from build123d import *

# Parameters (mm, degrees)
BOSS_EXTRUDE1_DEPTH  = 25.4
M3_CLEARANCE_HOLE1_D = 3.2
FILLET1_R            = 3


with BuildPart() as part:
    # Sketch1 → Boss-Extrude1 (new body)
    with BuildSketch(Plane(origin=(0, 0, 0), x_dir=(1, 0, 0), z_dir=(0, 1, 0))):
        with BuildLine():
            Line((-20, -20), (-9, -20))
            Line((-9, -20), (-9, -10.723805295))
            ThreePointArc((-9, -10.723805295), (0, 14), (9, -10.723805295))
            Line((9, -10.723805295), (9, -20))
            Line((9, -20), (20, -20))
            Line((20, -20), (20, 20))
            Line((20, 20), (-20, 20))
            Line((-20, 20), (-20, -20))
        make_face()
    extrude(amount=-BOSS_EXTRUDE1_DEPTH)

    # M3 Clearance Hole1 (through all)
    with Locations(Plane(origin=(-15.5, 0, -15.5), x_dir=(0, 0, 1), z_dir=(0, 1, 0))):
        with Locations((0, 0), (0, 31), (31, 31), (31, 0)):
            Hole(M3_CLEARANCE_HOLE1_D / 2)

    # Fillet1
    fillet1_edges = [part.edges().sort_by_distance(p)[0] for p in [
        (-9, -12.7, 10.723805295),
        (-9, -12.7, 20),
        (-20, -12.7, 20),
        (-20, -12.7, -20),
        (20, -12.7, -20),
        (20, -12.7, 20),
        (9, -12.7, 20),
        (9, -12.7, 10.723805295),
    ]]
    fillet(fillet1_edges, radius=FILLET1_R)


solid = part.part
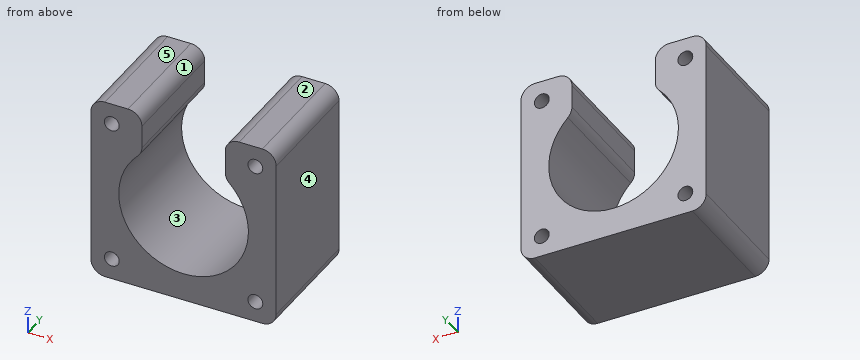
Could you check a few things on this model? Use its own coordinates, in mm. Face numbers are marked on the shaded views. A direction names the side the tool comes from. Give positions to 0.01 mm unless a question says otherwise; leave off trailing zeros. Write each loop counter-clockwise with the first axis right and the second up, starting at its lowest first coordinate (ties: lowest second). Pieces come first, ordered by that corner, then holes. Notation, with made-up numbers: (17, 36) -> (35, 36) arc R15 cw to (35, 46) -> close; hole circle Ø7 at (23, 4). An arc over 180 degrees is marked (long way). Answer as a JSON object with one key per item and string values.
Q1. Suppose I cut it at D-D on y = -12.25. Write out the boundary of the cut face in (x, z).
Taken from the geometry:
{"outline": "(-20, -17) arc R3 ccw to (-17, -20) -> (17, -20) arc R3 ccw to (20, -17) -> (20, 17) arc R3 ccw to (17, 20) -> (12, 20) arc R3 ccw to (9, 17) -> (9, 12.04) arc R3 ccw to (9.88, 9.92) arc R14 cw (long way) to (-9.88, 9.92) arc R3 ccw to (-9, 12.04) -> (-9, 17) arc R3 ccw to (-12, 20) -> (-17, 20) arc R3 ccw to (-20, 17) -> close; hole circle Ø3.2 at (-15.5, -15.5); hole circle Ø3.2 at (-15.5, 15.5); hole circle Ø3.2 at (15.5, -15.5); hole circle Ø3.2 at (15.5, 15.5)"}
Q2. Suppose I cut it at A-A on z = -15.5. Write out the boundary of the cut face in (x, y).
Taken from the geometry:
{"outline": "(-20, -25.4) -> (-17.1, -25.4) -> (-17.1, 0) -> (-20, 0) -> close; (-13.9, -25.4) -> (13.9, -25.4) -> (13.9, 0) -> (-13.9, 0) -> close; (17.1, -25.4) -> (20, -25.4) -> (20, 0) -> (17.1, 0) -> close"}
Q3. We'd pull the mould along X, two halves only. Please class the marked faces 3, 4 and 5: released by +X, released by -X, zero draft, split by the parting line, or undercut.
Taken from the geometry:
{"face 3": "undercut", "face 4": "released by +X", "face 5": "zero draft"}
Q4. Which directions (+Z, -Z, +X, -X, +Y, -Y) give clear straight access to the entire face, cutting with the end or side of a thin tool? Please do the marked faces 1 and 2.
Taken from the geometry:
{"face 1": "+Z, +Y, -Y", "face 2": "+Z, +X, -X, +Y, -Y"}
Q5. Suppose I cut it at B-B on x = 15.5. Write out the boundary of the cut face in (y, z).
Taken from the geometry:
{"outline": "(-25.4, -20) -> (0, -20) -> (0, -17.1) -> (-25.4, -17.1) -> close; (-25.4, -13.9) -> (0, -13.9) -> (0, 13.9) -> (-25.4, 13.9) -> close; (-25.4, 17.1) -> (0, 17.1) -> (0, 20) -> (-25.4, 20) -> close"}
Q6. Please list where these lines run through material, in increasing order: L1, parallel to Z at x = -15, y = -14.25; L2, parallel to X at y = -10.25, z = 13; L3, parallel to Z at x = 0, y = -13.25.
Taken from the geometry:
{"L1": "z = -20 to -17.02, -13.98 to 13.98, 17.02 to 20", "L2": "x = -20 to -9, 9 to 20", "L3": "z = -20 to -14"}
Q7. Suppose I cut it at C-C on z = 0. Write out the boundary of the cut face in (x, y), then the cut area to 3 significant figures.
Taken from the geometry:
{"outline": "(-20, -25.4) -> (-14, -25.4) -> (-14, 0) -> (-20, 0) -> close; (14, -25.4) -> (20, -25.4) -> (20, 0) -> (14, 0) -> close", "area": "305 mm²"}
